Part model, mm, in its own coordinate system. Face numbers are marked on the shaded views. Give positions to 0.01 mm unless a question says otherwise; leave off trailing zeros. Order: outer loops, then holes, each group sorted by start corner. A loop starts at its lowest first (then second) coordinate and runs counter-clockwise, first axis right, second up. Notation, with made-up numbers: (-16, -4.75) -> (31, -4.75) arc R10 ccw to (31, 5.25) -> close; hole circle Ø3 at (-15.5, 66.25). An arc over 180 degrees is marked (long way). Write item = value, one per line. Start each with the question number.
Item 1: Pull direction Y, two halves, no side cores. Call the marked faces 1, 2, 3 and 4: +Y half, -Y half, draft (parallel to the pull), parting line (faces both ways), or undercut.
Item 2: Flat gauge pins, fed straight in: P1, Ø2, axis at y = 167.5, z = 4.5, coming from the +X side; P2, Ø1.5, axis at y = 155, z = 2.5, coming from the -X side; P3, Ø1, axis at y = 151.5, z = 3, coming from the -X side. Where does each tip first touch, or does it go through?
Item 3: Band-saw the part on A-A on z = 3.75. Write the cut outline in (x, y) (3 decimals).
Item 4: Band-saw the part on B-B on x = 31.5. Write the cut outline in (y, z).
Item 5: Band-saw the part on C-C on y = 168.25. Write the cut outline in (x, z), plus the area to 3 significant figures.
Item 6: Drill centre lines: line 1 along X through (y, z) = (167, 3.5); line 2 along X through (y, z) = (170.75, 0.75); line 3 along X through (y, z) = (162.75, 5). Where is each one in solid material? Low to high.
Item 7: Band-saw the part on D-D on x = 0. Write the cut outline in (y, z).
```python
from build123d import *

# Parameters (mm, degrees)
BOSS_EXTRUDE2_DEPTH = 6.35


with BuildPart() as part:
    # Sketch1 → Boss-Extrude2 (new body)
    with BuildSketch(Plane.XY):
        with BuildLine():
            Line((37.717239544, 147.658964649), (35.965487423, 153.043027332))
            Line((35.965487423, 153.043027332), (33.550115758, 152.257164929))
            Line((33.550115758, 152.257164929), (30.406666146, 161.918651592))
            Line((30.406666146, 161.918651592), (32.822037812, 162.704513995))
            Line((32.822037812, 162.704513995), (29.806543337, 171.972726708))
            Line((29.806543337, 171.972726708), (22.86, 171.972726708))
            ThreePointArc((22.86, 171.972726708), (15.875, 164.987726708), (8.89, 171.972726708))
            Line((8.89, 171.972726708), (-8.89, 171.972726708))
            ThreePointArc((-8.89, 171.972726708), (-15.875, 164.987726708), (-22.86, 171.972726708))
            Line((-22.86, 171.972726708), (-29.806543337, 171.972726708))
            Line((-29.806543337, 171.972726708), (-32.822037812, 162.704513995))
            Line((-32.822037812, 162.704513995), (-30.406666146, 161.918651592))
            Line((-30.406666146, 161.918651592), (-33.550115758, 152.257164929))
            Line((-33.550115758, 152.257164929), (-35.965487423, 153.043027332))
            Line((-35.965487423, 153.043027332), (-37.717239544, 147.658964649))
            ThreePointArc((-37.717239544, 147.658964649), (0, 152.4), (37.717239544, 147.658964649))
        make_face()
    extrude(amount=BOSS_EXTRUDE2_DEPTH)


solid = part.part
```
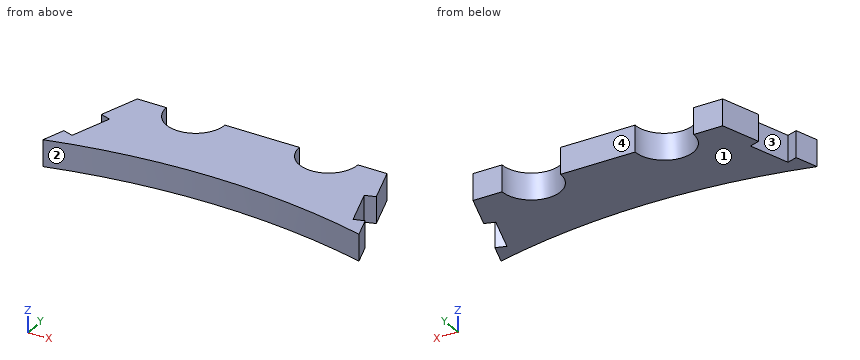
Values found:
q1.face_1 = draft
q1.face_2 = -Y half
q1.face_3 = undercut
q1.face_4 = +Y half
q2.P1 = 31.59
q2.P2 = -32.9
q2.P3 = -36.63
q3.outline = (-37.717, 147.659) arc R152.4 cw to (37.717, 147.659) -> (35.965, 153.043) -> (33.55, 152.257) -> (30.407, 161.919) -> (32.822, 162.705) -> (29.807, 171.973) -> (22.86, 171.973) arc R6.985 cw to (8.89, 171.973) -> (-8.89, 171.973) arc R6.985 cw to (-22.86, 171.973) -> (-29.807, 171.973) -> (-32.822, 162.705) -> (-30.407, 161.919) -> (-33.55, 152.257) -> (-35.965, 153.043) -> close
q4.outline = (149.11, 0) -> (158.56, 0) -> (158.56, 6.35) -> (149.11, 6.35) -> close; (162.27, 0) -> (166.77, 0) -> (166.77, 6.35) -> (162.27, 6.35) -> close
q5.outline = (-31.02, 0) -> (-21.79, 0) -> (-21.79, 6.35) -> (-31.02, 6.35) -> close; (-9.96, 0) -> (9.96, 0) -> (9.96, 6.35) -> (-9.96, 6.35) -> close; (21.79, 0) -> (31.02, 0) -> (31.02, 6.35) -> (21.79, 6.35) -> close
q5.area = 244 mm^2
q6.line_1 = -31.42 to -20.78, -10.97 to 10.97, 20.78 to 31.42
q6.line_2 = -30.2 to -22.75, -9 to 9, 22.75 to 30.2
q6.line_3 = -32.81 to 32.81
q7.outline = (152.4, 0) -> (171.97, 0) -> (171.97, 6.35) -> (152.4, 6.35) -> close
